from build123d import *

# Parameters (mm, degrees)
PAD026_DEPTH         = 16
SKETCH047_W          = 36.5505813425
SKETCH047_H          = 33
PAD027_DEPTH         = 16
SKETCH049_W          = 27
SKETCH049_H          = 5
PAD028_DEPTH         = 44.6
SKETCH048_W          = 33.1432370811
SKETCH048_H          = 35
POCKET031_DEPTH      = 16
SKETCH062_R          = 7
PAD029_DEPTH         = 40
SKETCH063_R          = 4
POCKET032_DEPTH      = 42
SKETCH065_R          = 5.1
POCKET033_DEPTH      = 33
SKETCH067_R          = 27
POCKET034_DEPTH      = 16
POCKET034_DEPTH_BACK = 16
POCKET050_DEPTH      = 23
PAD044_DEPTH         = 16
PAD045_DEPTH         = 26
PAD045_DEPTH_BACK    = 1
PAD046_DEPTH         = 26
PAD046_DEPTH_BACK    = 1
SKETCH099_R          = 1.5
POCKET051_DEPTH      = 5
SKETCH068_W          = 20.6
SKETCH068_H          = 23
POCKET052_DEPTH      = 7
SKETCH070_R          = 4
POCKET053_DEPTH      = 16


with BuildPart() as part:
    # Sketch045 → Pad026 (new body)
    with BuildSketch(Plane.XY):
        with BuildLine():
            ThreePointArc((16.6337166542, -23.7554092844), (0, 29), (-16.6337166542, -23.7554092844))
            Line((-16.6337166542, -23.7554092844), (16.6337166542, -23.7554092844))
        make_face()
    extrude(amount=PAD026_DEPTH)

    # Sketch047 → Pad027 (join)
    with BuildSketch(Plane.XY):
        with Locations((-1.6415607576, -40.2554)):
            Rectangle(SKETCH047_W, SKETCH047_H)
    extrude(amount=PAD027_DEPTH)

    # Sketch049 → Pad028 (join)
    with BuildSketch(Plane(origin=(-19.9168514289, 0, 0), x_dir=(0, -1, 0), z_dir=(-1, 0, 0))):
        with Locations((43.2554, 10.5)):
            Rectangle(SKETCH049_W, SKETCH049_H)
    extrude(amount=PAD028_DEPTH)

    # Sketch048 → Pocket031 (cut)
    with BuildSketch(Plane.XY):
        with Locations((1.7499799388, -41.2554)):
            Rectangle(SKETCH048_W, SKETCH048_H)
    extrude(amount=POCKET031_DEPTH, mode=Mode.SUBTRACT)

    # Sketch062 → Pad029 (join)
    with BuildSketch(Plane.YZ):
        with Locations((-17.7554, 0)):
            Circle(SKETCH062_R)
    extrude(amount=PAD029_DEPTH)

    # Sketch063 → Pocket032 (cut)
    with BuildSketch(Plane.YZ):
        with Locations((-17.7554, 0)):
            Circle(SKETCH063_R)
    extrude(amount=POCKET032_DEPTH, mode=Mode.SUBTRACT)

    # Sketch065 → Pocket033 (cut)
    with BuildSketch(Plane.YZ):
        with Locations((-17.7554, 0)):
            Circle(SKETCH065_R)
    extrude(amount=POCKET033_DEPTH, mode=Mode.SUBTRACT)

    # Sketch067 → Pocket034 (cut, two sides)
    with BuildSketch(Plane(origin=(0, 0, 0), x_dir=(1, 0, 0), z_dir=(0, 0, -1))) as pocket034_sk:
        Circle(SKETCH067_R)
    extrude(amount=-POCKET034_DEPTH, mode=Mode.SUBTRACT)
    extrude(pocket034_sk.sketch, amount=POCKET034_DEPTH_BACK, mode=Mode.SUBTRACT)

    # Sketch069 → Pocket050 (cut)
    with BuildSketch(Plane.XY.offset(16)):
        with BuildLine():
            ThreePointArc((21.7394688414, -34.7619834661), (34.6744517723, -21.8788115374), (40.7345717373, -4.6577532545))
            Line((40.7345717373, -4.6577532545), (77.483603, -4.6577532545))
            Line((77.483603, -4.6577532545), (77.483603, -35.651409))
            Line((21.7394688414, -34.7619834661), (77.483603, -35.651409))
        make_face()
    extrude(amount=-POCKET050_DEPTH, mode=Mode.SUBTRACT)

    # Sketch072 → Pad044 (join)
    with BuildSketch(Plane(origin=(0, 0, 0), x_dir=(1, 0, 0), z_dir=(0, 0, -1))):
        Polygon((-19.92, 25.478123), (-19.92, 19.578123), (-15.1, 25.478123), align=None)
    extrude(amount=-PAD044_DEPTH)

    # Sketch101 → Pad045 (join, two sides)
    with BuildSketch(Plane.XZ.offset(55.7554)) as pad045_sk:
        with BuildLine():
            ThreePointArc((-23.0890778045, 12.9959643316), (-20.9165956412, 13.739198554), (-19.9059643934, 15.8009212171))
            Line((-19.9059643933, 15.8009212171), (-17.161644, 10.394013))
            Line((-23.0890778045, 12.9959643316), (-17.161644, 10.394013))
        make_face()
    extrude(amount=-PAD045_DEPTH)
    extrude(pad045_sk.sketch, amount=PAD045_DEPTH_BACK)

    # Sketch100 → Pad046 (join, two sides)
    with BuildSketch(Plane.XZ.offset(55.7554)) as pad046_sk:
        with BuildLine():
            ThreePointArc((-19.6511636096, 2.9781881147), (-21.3108750101, 7.3106091304), (-25.5643652158, 9.1632652939))
            Line((-25.564365, 9.163265), (-16.937498, 9.628842))
            Line((-19.651164, 2.978188), (-16.937498, 9.628842))
        make_face()
    extrude(amount=-PAD046_DEPTH)
    extrude(pad046_sk.sketch, amount=PAD046_DEPTH_BACK)

    # Sketch099 → Pocket051 (cut)
    with BuildSketch(Plane(origin=(0, 0, 8), x_dir=(1, 0, 0), z_dir=(0, 0, -1))):
        with Locations((-45.92, 37.2554)):
            Circle(SKETCH099_R)
        with Locations((-45.92, 50.2554)):
            Circle(SKETCH099_R)
        with Locations((-42.92, 43.7554)):
            Circle(SKETCH099_R)
    extrude(amount=-POCKET051_DEPTH, mode=Mode.SUBTRACT)

    # Sketch068 (on DatumPlane) → Pocket052 (cut)
    with BuildSketch(Plane(origin=(24.3662700863, -13, 0), x_dir=(-0.5, -0.8660254038, 0), z_dir=(-0.6123724357, 0.3535533906, -0.7071067812))):
        with Locations((6.74, -3)):
            Rectangle(SKETCH068_W, SKETCH068_H)
    extrude(amount=POCKET052_DEPTH, mode=Mode.SUBTRACT)

    # Sketch070 → Pocket053 (cut)
    with BuildSketch(Plane(origin=(0, 0, 0), x_dir=(1, 0, 0), z_dir=(0, 0, -1))):
        with Locations((-13.85, 23)):
            Circle(SKETCH070_R)
    extrude(amount=-POCKET053_DEPTH, mode=Mode.SUBTRACT)


solid = part.part
Geometry check sheet. Reference: the model listing, model coordinates, mm. A direction names the side the tool comes from. Coordinates: 2 decimals unless noted, no trailing zeros. Order: outer loops, then holes, each group sorted by start corner. A loop starts at its lowest first (then second) coordinate and runs counter-clockwise, first axis right, second up. Notation, with made-up numbers: M 37,-36.75 L 96,-36.75 A23 ccw 96,-10.75 Z; hole C -17.75,76.5 d5. An arc over 180 degrees is marked long. Use CSV: the item, a comma, the result in double quotes.
Item 1: Cross-section at C-C on y = -40. Record the cut outline in (x, z).
Returned:
outline,"M -64.52,8 L -22.1,8 A6 cw -19.92,4.94 L -19.92,0 L -14.82,0 L -14.82,16 L -19.92,16 L -19.92,15.67 A3 cw -22.66,13 L -64.52,13 Z"
Item 2: Cross-section at A-A on x = -45.92. Record the cut outline in (y, z).
Returned:
outline,"M -56.76,8 L -51.76,8 L -51.76,13 L -56.76,13 Z; M -48.76,8 L -38.76,8 L -38.76,13 L -48.76,13 Z; M -35.76,8 L -29.76,8 L -29.76,13 L -35.76,13 Z"
Item 3: Tool access check on faces 1 (the cylindrical face through (26.19, -21.51, 3.45)), 2 (the cylindrical face through (-20.83, -43.07, 13.82)), 3 (the flat face through (-42, -29.755, 11)), 4 (the cylindrical face through (-17.554, -24.509, 7.888)), 5 (the flat face through (-14.822, -42, 8)). Record the directions out of +Z, -Z, +X, -X, +Y, -Y that give a thin tool (end or side, any length) a straight path to the whole face; none if there is none.
Returned:
face 1,"none"
face 2,"+Z, -X, -Y"
face 3,"+Z, -Z, -X"
face 4,"+Z, -Z"
face 5,"+Z, -Z, +X, -Y"
Item 4: Gauge pin test, flat ends, axial feed: pin 1 Ø5 at (x, y) = (-44.5, -36) entering from -Z; pin 2 Ø8 at (y, z) = (-10.5, 4) entering from +X; pin 3 Ø6.5 at (y, z) = (-17.76, 0) entering from -X; pin 4 Ø9 at (y, z) = (-17.76, 0) entering from +X. Record the tip position at first contact, or that the pin passes through.
Returned:
pin 1,"stops at z = 8"
pin 2,"stops at x = 39.56"
pin 3,"stops at x = -25.11"
pin 4,"stops at x = 38.8"
Item 5: Cross-section at B-B on y = 0. Record the cut outline in (x, z), then the cut area to 3 significant figures.
Returned:
outline,"M -29,0 L -27,0 L -27,16 L -29,16 Z; M 27,0 L 29,0 L 29,16 L 27,16 Z"
area,"64.0 mm2"
Item 6: Thickness scan on line 1 along X through (y, z) = (0, 8.75); line 2 along Z through (x, y) = (-50, -44.5); line 3 along X through (y, z) = (-43, 4.5). Record the ranges inside material, lowest first.
Returned:
line 1,"x = -29 to -27, 27 to 29"
line 2,"z = 8 to 13"
line 3,"x = -19.92 to -14.82"
Item 7: Mould release check, pull along Y, two halves, no side actions. Record for faces 6 (the cylindrical face through (38.158, -14.998, 3.211)), 7 (the flat face through (-19.92, -23, 8)), 8 (the flat face through (-64.517, -43, 11)), 9 (the flat face through (25.87, -20.47, -5.04)): pulls with the +Y half, pulls with the -Y half, needs draft (parallel to the pull), parting line crosses it, or undercut.
Returned:
face 6,"pulls with the -Y half"
face 7,"undercut"
face 8,"needs draft"
face 9,"undercut"
